from build123d import *

# Parameters (mm, degrees)
SKETCH1_W               = 63.5
SKETCH1_H               = 83.82
BOSS_EXTRUDE1_DEPTH     = 19.05
SHELL1_T                = -2.54
CUT_EXTRUDE1_REACH      = 57.11
SKETCH2_R               = 17.399
FILLET4_R               = 6.35
CUT_EXTRUDE2_DEPTH      = 92.633822358
CUT_EXTRUDE2_DEPTH_BACK = 92.633822358
SKETCH3_R               = 2.0955


with BuildPart() as part:
    # Sketch1 → Boss-Extrude1 (new body)
    with BuildSketch(Plane.XY):
        Rectangle(SKETCH1_W, SKETCH1_H)
    extrude(amount=BOSS_EXTRUDE1_DEPTH)

    # Shell1
    shell1_openings = [part.faces().sort_by_distance(p)[0] for p in [
        (0, 0, 19.05),
    ]]
    offset(amount=SHELL1_T, openings=shell1_openings, kind=Kind.INTERSECTION)

    # Sketch2 → Cut-Extrude1 (cut, up to next)
    with BuildSketch(Plane.XY.offset(2.54), mode=Mode.PRIVATE) as cut_extrude1_sk1:
        Circle(SKETCH2_R)
    cut_extrude1_tool1 = extrude(cut_extrude1_sk1.sketch, amount=-CUT_EXTRUDE1_REACH, mode=Mode.PRIVATE) & part.part
    add(cut_extrude1_tool1.solids().sort_by_distance((0, 0, 2.54))[0], mode=Mode.SUBTRACT)

    # Fillet4
    fillet4_edges = [part.edges().sort_by_distance(p)[0] for p in [
        (31.75, -41.91, 9.525),
        (-31.75, -41.91, 9.525),
        (-31.75, 41.91, 9.525),
        (31.75, 41.91, 9.525),
    ]]
    fillet(fillet4_edges, radius=FILLET4_R)

    # Sketch3 → Cut-Extrude2 (cut, two sides: drawn at the far end of the back side and taken through both)
    with BuildSketch(Plane(origin=(0, 41.91, 0), x_dir=(1, 0, 0), z_dir=(0, 1, 0)).offset(-CUT_EXTRUDE2_DEPTH_BACK)):
        with Locations(Location((0, -11.176, 0), (0, 0, 270))):
            Circle(SKETCH3_R)
    extrude(amount=CUT_EXTRUDE2_DEPTH + CUT_EXTRUDE2_DEPTH_BACK, mode=Mode.SUBTRACT)


solid = part.part
Could you check a few things on this model? Use its own coordinates, in mm. A direction names the side the tool comes from. Coordinates: 2 decimals unless noted, no trailing zeros. Order: outer loops, then holes, each group sorted by start corner. A loop starts at its lowest first (then second) coordinate and runs counter-clockwise, first axis right, second up.
Q1. Thinking about a two-plate mould opening in X: for faces 3 (the cylindrical face through (-29.94, -40, 9.66)), 4 (the cylindrical face through (-0.803, -40.658, 13.112)), 5 (the flat face through (0, -41.91, 7)), which applies, released by +X, released by -X, zero draft, split by the parting line, or undercut?
Q2. Suppose I cut it at A-A on z = 7.5. Please give me the cut outline in (x, y), and give its area (3 significant figures).
Q3. Which directions (+Z, -Z, +X, -X, +Y, -Y) give clear straight access to the entire face, cutting with the end or side of a thin tool? Please do faces 1 (the cylindrical face through (29.84, -40.1, 9.66)), 2 (the flat face through (-29.21, -1, 11)).
Q4. Please list where these lines run through material, in increasing order: L1, parallel to Y at x = 25, z = 7.5; L2, parallel to X at y = -27, z = 8.75; L3, parallel to Z at x = 0, y = 40.
Q5. Will this pin go through, and if not, where does the flat tip stop? pin 1 (4 mm diameter, centred on x = -6, y = -24, fed in from +Z).
Q6. Suppose I cut it at C-C on y = 0. Please give me the cut outline in (x, z).
Q7. Suppose I cut it at D-D on x = -14. Please give me the cut outline in (y, z).
Q8. Suppose I cut it at B-B on x = 0. Please give me the cut outline in (y, z).
Answer:
1. face 3: released by -X
1. face 4: undercut
1. face 5: zero draft
2. outline: (-31.75, -35.56) arc R6.35 ccw to (-25.4, -41.91) - (25.4, -41.91) arc R6.35 ccw to (31.75, -35.56) - (31.75, 35.56) arc R6.35 ccw to (25.4, 41.91) - (-25.4, 41.91) arc R6.35 ccw to (-31.75, 35.56) - close; hole (-29.21, -39.37) - (29.21, -39.37) - (29.21, 39.37) - (-29.21, 39.37) - close
2. area: 688 mm2
3. face 1: +Z, -Z, +X, -Y
3. face 2: +Z
4. L1: y = -41.91 to -39.37, 39.37 to 41.91
4. L2: x = -31.75 to -29.21, 29.21 to 31.75
4. L3: z = 0 to 9.08, 13.27 to 19.05
5. pin 1: stops at z = 2.54
6. outline: (-31.75, 0) - (-17.4, 0) - (-17.4, 2.54) - (-29.21, 2.54) - (-29.21, 19.05) - (-31.75, 19.05) - close; (17.4, 0) - (31.75, 0) - (31.75, 19.05) - (29.21, 19.05) - (29.21, 2.54) - (17.4, 2.54) - close
7. outline: (-41.91, 0) - (-10.33, 0) - (-10.33, 2.54) - (-39.37, 2.54) - (-39.37, 19.05) - (-41.91, 19.05) - close; (10.33, 0) - (41.91, 0) - (41.91, 19.05) - (39.37, 19.05) - (39.37, 2.54) - (10.33, 2.54) - close
8. outline: (-41.91, 0) - (-17.4, 0) - (-17.4, 2.54) - (-39.37, 2.54) - (-39.37, 9.08) - (-41.91, 9.08) - close; (-41.91, 13.27) - (-39.37, 13.27) - (-39.37, 19.05) - (-41.91, 19.05) - close; (17.4, 0) - (41.91, 0) - (41.91, 9.08) - (39.37, 9.08) - (39.37, 2.54) - (17.4, 2.54) - close; (39.37, 13.27) - (41.91, 13.27) - (41.91, 19.05) - (39.37, 19.05) - close
